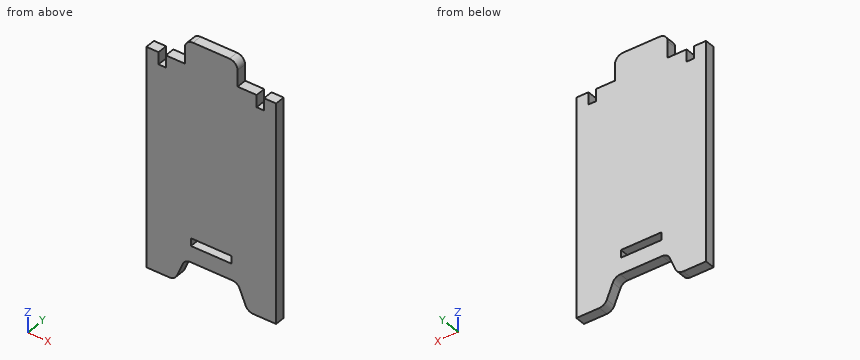
from build123d import *

# Parameters (mm, degrees)
F0_W     = 320
F0_H     = 600
F1_DEPTH = 25
F2_W     = 100
F2_H     = 19
F2_W_2   = 18
F2_H_2   = 30
F3_DEPTH = 25


with BuildPart() as f1:
    # F0 (on Front) → F1 (new body)
    with BuildSketch(Plane.XZ):
        Rectangle(F0_W, F0_H)
    extrude(amount=F1_DEPTH)

    # F2 (on face) → F3 (cut, through all)
    with BuildSketch(Plane.XZ.offset(25)):
        with BuildLine():
            Line((-160, 300), (-160, 240))
            Line((-160, 240), (-130, 240))
            Line((-130, 240), (-112, 240))
            Line((-112, 240), (-85, 240))
            Line((-85, 240), (-65, 240))
            Line((-65, 240), (-65, 260))
            Line((-65, 260), (-65, 280))
            ThreePointArc((-65, 280), (-59.142136, 294.142136), (-45, 300))
            Line((-45, 300), (-160, 300))
        make_face()
        with BuildLine():
            Line((130, 240), (160, 240))
            Line((160, 240), (160, 300))
            Line((160, 300), (45, 300))
            ThreePointArc((45, 300), (59.142136, 294.142136), (65, 280))
            Line((65, 280), (65, 260))
            Line((65, 260), (65, 240))
            Line((65, 240), (85, 240))
            Line((85, 240), (112, 240))
            Line((112, 240), (130, 240))
        make_face()
        with BuildLine():
            Line((-70.128205, -252.307692), (-84.871795, -287.692308))
            ThreePointArc((-84.871795, -287.692308), (-92.239329, -296.641006), (-103.333333, -300))
            Line((-103.333333, -300), (103.333333, -300))
            ThreePointArc((103.333333, -300), (92.239329, -296.641006), (84.871795, -287.692308))
            Line((84.871795, -287.692308), (70.128205, -252.307692))
            ThreePointArc((70.128205, -252.307692), (62.760671, -243.358994), (51.666667, -240))
            Line((51.666667, -240), (-51.666667, -240))
            ThreePointArc((-51.666667, -240), (-62.760671, -243.358994), (-70.128205, -252.307692))
        make_face()
        with Locations((0, -190.5)):
            Rectangle(F2_W, F2_H)
        with Locations((-121, 225)):
            Rectangle(F2_W_2, F2_H_2)
        with Locations((121, 225)):
            Rectangle(F2_W_2, F2_H_2)
    extrude(amount=-F3_DEPTH, mode=Mode.SUBTRACT)


solid = f1.part
The listing builds one solid part. Answer for the finished solid, in the listing's coordinates (mm). Give positions to 0.01 mm unless a question says otherwise; leave off trailing zeros. Write each loop counter-clockwise with the first axis right and the second up, starting at its lowest first coordinate (ties: lowest second). Pieces come first, ordered by that corner, then holes. Notation, with made-up numbers: (7, 49.5) - (59, 49.5) arc R23 cw to (59, 57.5) - close; hole circle Ø10 at (27, 40). An arc over 180 degrees is marked (long way). Use a Markdown table: item, result.
1. Section A-A on x = 9.5 is taken. Write down the section's boundary in (y, z).
Values follow:
| item | result |
|---|---|
| outline | (-25, -240) - (0, -240) - (0, -200) - (-25, -200) - close; (-25, -181) - (0, -181) - (0, 300) - (-25, 300) - close |
2. Section C-C on x = 78 is taken. Write down the section's boundary in (y, z).
Values follow:
| item | result |
|---|---|
| outline | (-25, -271.2) - (0, -271.2) - (0, 240) - (-25, 240) - close |
3. Each of these flat-tipped pins is pushed along its axis until it touches: P1, Ø9, axis at x = 122.5, y = -9.5, coming from the +Z side; P2, Ø3, axis at x = 103.5, z = -107.5, coming from the +Y side; P3, Ø12.5, axis at x = 3.5, y = -10, coming from the -Z side; P4, Ø7.5, axis at x = 144, y = -14.5, coming from the +Z side. Where does it stop, or does it pass through?
Values follow:
| item | result |
|---|---|
| P1 | stops at z = 210 |
| P2 | stops at y = 0 |
| P3 | stops at z = -240 |
| P4 | stops at z = 240 |
4. Section D-D on z = 257.5 is taken. Write down the section's boundary in (x, y), plus the area to 3 significant figures.
Values follow:
| item | result |
|---|---|
| outline | (-65, -25) - (65, -25) - (65, 0) - (-65, 0) - close |
| area | 3,250 mm² |
5. Find the intervals of material crossed by probe 1 along Z at (x, y) = (41, -2.25); probe 2 along Z at (x, y) = (119, -13); probe 3 along Z at (x, y) = (131.5, -12.75), in increasing order. Write a range as from..to.
Values follow:
| item | result |
|---|---|
| probe 1 | z = -240..-200, -181..300 |
| probe 2 | z = -300..210 |
| probe 3 | z = -300..240 |
